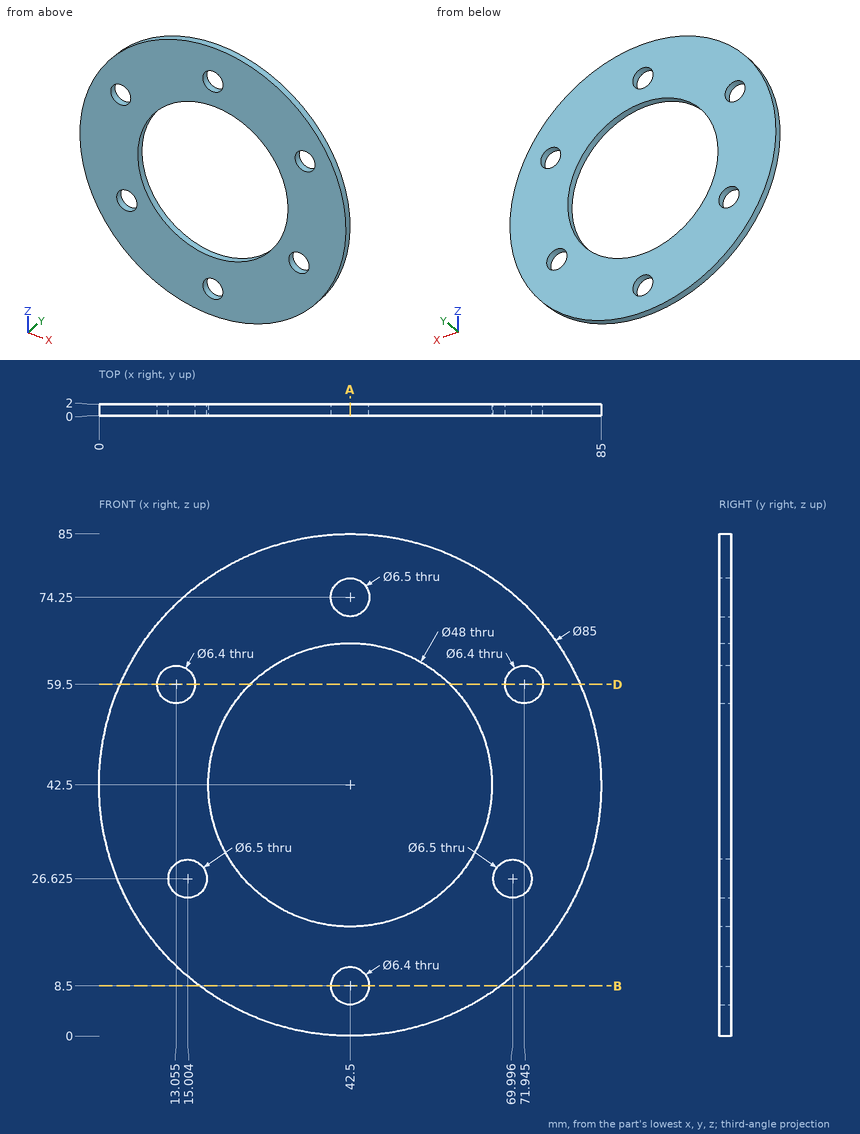
Geometry check sheet. Reference: drawing and pictorial views, mm from the part's lowest x, y, z. Coordinates: 2 decimals unless noted, no trailing zeros. Order: outer loops, then holes, each group sorted by start corner. A loop starts at its lowest first (then second) coordinate and runs counter-clockwise, first axis right, second up.
Item 1: Section check D-D (z = 59.5). Enter the section's corners in (x, y) (1 decimal).
Item 2: Scan lines: line 1 along X through (y, z) = (1.85, 57.5) (1 decimal); line 2 along X through (y, z) = (1.6, 59.5) (1 decimal); line 3 along X through (y, z) = (0.75, 42.5). Record each from-to range of solid material in increasing order.
Item 3: Section check A-A (x = 42.5). Enter the section's corners in (y, z).
Item 4: Depth check by flat-ended pin: pin 1 (8.5 mm diameter, centred on x = 42.5, z = 74.25, fed in from -Y); pin 2 (1 mm diameter, centred on y = 1, z = 59.5, fed in from +X). Enter the tip coordinate at first touch or a pass-through.
Item 5: Section check B-B (z = 8.5). Enter the section's corners in (x, y).
Check sheet entries:
1. outline: (3.5, 0) - (9.9, 0) - (9.9, 2) - (3.5, 2) - close; (16.3, 0) - (25.6, 0) - (25.6, 2) - (16.3, 2) - close; (59.4, 0) - (68.7, 0) - (68.7, 2) - (59.4, 2) - close; (75.1, 0) - (81.5, 0) - (81.5, 2) - (75.1, 2) - close
2. line 1: x = 2.7 to 10.6, 15.6 to 23.8, 61.2 to 69.4, 74.4 to 82.3
2. line 2: x = 3.5 to 9.9, 16.3 to 25.6, 59.4 to 68.7, 75.1 to 81.5
2. line 3: x = 0 to 18.5, 66.5 to 85
3. outline: (0, 0) - (2, 0) - (2, 5.3) - (0, 5.3) - close; (0, 11.7) - (2, 11.7) - (2, 18.5) - (0, 18.5) - close; (0, 66.5) - (2, 66.5) - (2, 71) - (0, 71) - close; (0, 77.5) - (2, 77.5) - (2, 85) - (0, 85) - close
4. pin 1: stops at y = 0
4. pin 2: stops at x = 81.67
5. outline: (17, 0) - (39.3, 0) - (39.3, 2) - (17, 2) - close; (45.7, 0) - (68, 0) - (68, 2) - (45.7, 2) - close
